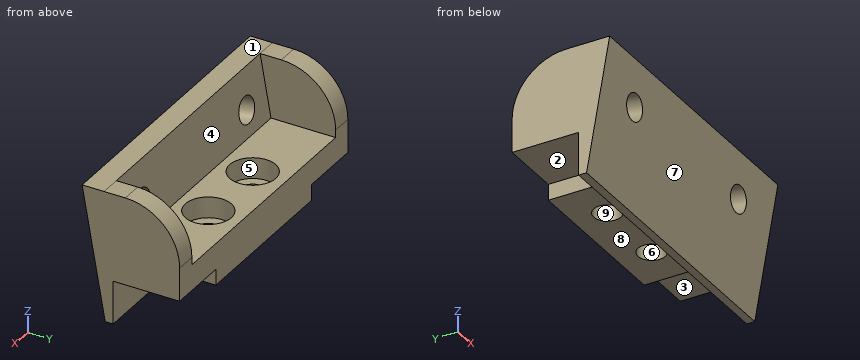
from build123d import *

# Parameters (mm, degrees)
PAD004_DEPTH    = 55
SKETCH007_R     = 2.6
POCKET_DEPTH    = 10
SKETCH005_R     = 2.5
POCKET002_DEPTH = 5
SKETCH008_R     = 4.4
POCKET003_DEPTH = 5
PAD005_DEPTH    = 4
PAD006_DEPTH    = 4
POCKET005_DEPTH = 12.7


with BuildPart() as part:
    # Sketch004 → Pad004 (new body)
    with BuildSketch(Plane.YZ):
        Polygon((-1.516354, -5.192676), (-5.924528, 19.807324), (-1.724528, 19.807324), (0.357421, 8), (12.7, 8), (12.7, 0), (0, 0), (0, -5.192676), align=None)
    extrude(amount=PAD004_DEPTH)

    # Sketch007 → Pocket (cut)
    with BuildSketch(Plane.XY):
        with Locations((20.25, 6.35)):
            Circle(SKETCH007_R)
        with Locations((34.75, 6.35)):
            Circle(SKETCH007_R)
    extrude(amount=POCKET_DEPTH, mode=Mode.SUBTRACT)

    # Sketch005 → Pocket002 (cut)
    with BuildSketch(Plane(origin=(0, 2, 0), x_dir=(-1, 0, 0), z_dir=(0, 0.984808, 0.173648))):
        with Locations((-44.475514, 12.925289)):
            Circle(SKETCH005_R)
        with Locations((-10.524486, 12.925289)):
            Circle(SKETCH005_R)
    extrude(amount=-POCKET002_DEPTH, mode=Mode.SUBTRACT)

    # Sketch008 → Pocket003 (cut)
    with BuildSketch(Plane.XY.offset(4)):
        with Locations((20.25, 6.35)):
            Circle(SKETCH008_R)
        with Locations((34.75, 6.35)):
            Circle(SKETCH008_R)
    extrude(amount=POCKET003_DEPTH, mode=Mode.SUBTRACT)

    # Sketch009 → Pad005 (join)
    with BuildSketch(Plane.YZ):
        with BuildLine():
            Line((12.7, 8), (0.357421, 8))
            Line((0.357421, 8), (-1.724529, 19.807325))
            Line((-1.724529, 19.807325), (2.337742, 19.807325))
            ThreePointArc((12.7, 9.445067), (9.664965, 16.77229), (2.337742, 19.807325))
            Line((12.7, 9.445067), (12.7, 8))
        make_face()
    extrude(amount=PAD005_DEPTH)

    # Sketch010 → Pad006 (join)
    with BuildSketch(Plane.YZ.offset(55)):
        with BuildLine():
            Line((12.7, 8), (0.357421, 8))
            Line((0.357421, 8), (-1.724529, 19.807325))
            Line((-1.724529, 19.807325), (2.337742, 19.807325))
            ThreePointArc((12.7, 9.445067), (9.664965, 16.77229), (2.337742, 19.807325))
            Line((12.7, 9.445067), (12.7, 8))
        make_face()
    extrude(amount=-PAD006_DEPTH)

    # Sketch012 (on Face10 of Pad006) → Pocket005 (cut)
    with BuildSketch(Plane.ZX.offset(12.7)):
        Polygon((0, 43.184493), (3.048737, 43.184493), (3.048737, 55), (-3.047035, 55), (-3.047035, 0), (0, 0), (3.048737, 0), (3.048737, 11.815507), (0, 11.815507), align=None)
    extrude(amount=-POCKET005_DEPTH, mode=Mode.SUBTRACT)


with BuildPart() as part_1:
    # Body004 placement: moved
    add(part.part.moved(Location((12.5222, -6.2992, 12.7254))))


solid = part_1.part
Can you work these out from the model? Positions are in its coordinate system, mm. Face numbers are marked on the shaded views. A direction names the side the tool comes from. Coordinates: 2 decimals unless noted, no trailing zeros. Write each loop counter-clockwise with the first axis right and the second up, starting at its lowest first coordinate (ties: lowest second). Pieces come first, ordered by that corner, then holes. Notation, with made-up numbers: (60.5, 81) -> (95.5, 81) arc R27 ccw to (95.5, 98) -> close; hole circle Ø7 at (62.25, 56). An arc over 180 degrees is marked (long way). Answer as CSV lines item,"result".
1) If we section it at C-C on x = 39: Please give me the cut outline in (y, z), then the cut area to 3 significant figures.
Check result:
outline,"(-12.22, 32.53) -> (-7.82, 7.53) -> (-6.3, 7.53) -> (-6.3, 12.73) -> (6.4, 12.73) -> (6.4, 20.73) -> (-5.94, 20.73) -> (-8.02, 32.53) -> close"
area,"187 mm²"
2) If we section it at B-B on x = 21.5: Please give me the cut outline in (y, z).
Check result:
outline,"(-12.22, 32.53) -> (-11.18, 26.63) -> (-7.11, 27.35) -> (-8.02, 32.53) -> close; (-10.5, 22.76) -> (-7.82, 7.53) -> (-6.3, 7.53) -> (-6.3, 15.77) -> (6.4, 15.77) -> (6.4, 20.73) -> (-5.94, 20.73) -> (-6.43, 23.48) -> close"
3) On a 3-axis mill with a long thin cutter (end or side, diameter ignored), from which of +Z, -Z, +X, -X, +Y, -Y can I reach the whole of each face in a straight line? I mean the marked faces 1, 2, 3, 4 and 5. Say none if no direction works.
Check result:
face 1,"+Z, +X, -X, +Y, -Y"
face 2,"-Z, -X, +Y"
face 3,"-Z, +X, +Y"
face 4,"+Z, +Y"
face 5,"+Z"
4) If we mould it in two halves opening along Y, with no side actions, what happens to the marked faces 6, 7, 8 and 9? For each: +Y half, -Y half, draft (parallel to the pull), parting line (faces both ways), or undercut.
Check result:
face 6,"undercut"
face 7,"-Y half"
face 8,"draft"
face 9,"undercut"
5) Will these pins go through, and if not, where does the flat tip stop? P1, Ø4, axis at x = 39, y = 1, coming from the -Z side; P2, Ø1.5, axis at x = 24.5, z = 27.5, coming from the +Y side; P3, Ø1.5, axis at x = 22, y = -5, coming from the -Z side.
Check result:
P1,"z = 12.73"
P2,"y = -7.04"
P3,"z = 15.77"
6) If we section it at A-A on y = 1: Please give me the cut outline in (x, z).
Check result:
outline,"(12.52, 15.77) -> (24.34, 15.77) -> (24.34, 12.73) -> (30.35, 12.73) -> (30.35, 16.73) -> (28.48, 16.73) -> (28.48, 20.73) -> (16.52, 20.73) -> (16.52, 31.27) -> (12.52, 31.27) -> close; (35.19, 12.73) -> (44.85, 12.73) -> (44.85, 16.73) -> (42.98, 16.73) -> (42.98, 20.73) -> (37.07, 20.73) -> (37.07, 16.73) -> (35.19, 16.73) -> close; (49.69, 12.73) -> (55.71, 12.73) -> (55.71, 15.77) -> (67.52, 15.77) -> (67.52, 31.27) -> (63.52, 31.27) -> (63.52, 20.73) -> (51.57, 20.73) -> (51.57, 16.73) -> (49.69, 16.73) -> close"
7) If I drill on line 1 (X direction, y = 0, z = 14); line 2 (X direction, y = -6.5, z = 29.25); line 3 (Y direction, x = 34, z = 20.5), over which ranges is the centre line in solid material (lowest first)? Write a range as from..to.
Check result:
line 1,"24.34..30.17, 35.37..44.67, 49.87..55.71"
line 2,"12.52..16.52, 63.52..67.52"
line 3,"-10.1..-4.17, 4.28..6.4"
8) If we section it at D-D on z = 28.75: Please give me the cut outline in (x, y), then the cut area to 3 significant figures.
Check result:
outline,"(12.52, -11.56) -> (67.52, -11.56) -> (67.52, 4.04) -> (63.52, 4.04) -> (63.52, -7.36) -> (16.52, -7.36) -> (16.52, 4.04) -> (12.52, 4.04) -> close"
area,"322 mm²"
